Geometry check sheet. Reference: the model listing, model coordinates, mm. Face numbers are marked on the shaded views. A direction names the side the tool comes from. Give positions to 0.01 mm unless a question says otherwise; leave off trailing zeros. Order: outer loops, then holes, each group sorted by start corner. A loop starts at its lowest first (then second) coordinate and runs counter-clockwise, first axis right, second up. Notation, with made-up numbers: M -10,36 L 44,36 A16 cw 44,42 Z; hole C 15,77.25 d5. An arc over 180 degrees is marked long. Answer as CSV lines item,"result". Start each with the question number.
Q1. Section check A-A, the plane y = 24.5. Record the boundary of the cut face in (x, z).
Q2. Go/stop test with flat-tipped pins: pin 1 (1.5 mm diameter, centred on y = 56.5, z = 43.5, fed in from -X); pin 2 (5 mm diameter, centred on x = -24, y = 23.5, fed in from -Z); pin 3 (3 mm diameter, centred on x = 53, y = 30.5, fed in from +Z). Record where each tip stops, or that it passes through.
Q3. Section check D-D, the plane y = 62. Record the boundary of the cut face in (x, z), then the cut area to 3 significant figures.
Q4. Section check B-B, the plane x = 23.5. Record the boundary of the cut face in (y, z), then the cut area to 3 significant figures.
Q5. Set-up check for the marked faces 1, 2 and 3: record each of +Z, -Z, +X, -X, +Y, -Y from which the full face is reachable in a straight line by a thin tool's end or side.
Q6. Thickness scan on line 1 (X direction, y = 8, z = 107); line 2 (Z direction, x = -91, y = 5); line 3 (X direction, y = 18, z = 128). Record the ranges inside material, lowest first.
Q7. Section check C-C, the plane z = 39.5. Record the boundary of the cut face in (x, y).
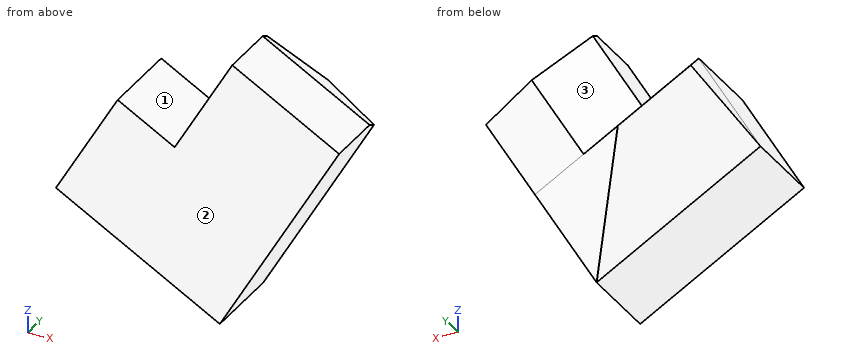
```python
from build123d import *

# Parameters (mm, degrees)
EXTRUDE1_DEPTH     = 50
EXTRUDE2_DEPTH     = 115
EXTRUDE3_DEPTH     = 105
CUT_EXTRUDE1_DEPTH = 155
CUT_EXTRUDE2_DEPTH = 75


with BuildPart() as part:
    # Sketch1 → Extrude1 (new body)
    with BuildSketch(Plane(origin=(0, 0, 0), x_dir=(1, 0, 0), z_dir=(0, 1, 0))):
        Polygon((0, 0), (72.5, -125.573683549), (7.548094716, -163.073683549), (-27.451905284, -102.451905284), (-62.092921435, -122.451905284), (-99.592921435, -57.5), align=None)
    extrude(amount=EXTRUDE1_DEPTH)

    # Sketch2 → Extrude2 (add)
    with BuildSketch(Plane(origin=(-99.592921435, 0, 57.5), x_dir=(0.5, 0, 0.866025404), z_dir=(-0.866025404, 0, 0.5))):
        Polygon((75, 50), (0, 50), (37.5, 94.690759722), align=None)
    extrude(amount=-EXTRUDE2_DEPTH)

    # Sketch3 → Extrude3 (add)
    with BuildSketch(Plane(origin=(72.5, 0, 125.573683549), x_dir=(0.866025404, 0, -0.5), z_dir=(0.5, 0, 0.866025404))):
        Polygon((0, 50), (-75, 50), (-37.5, 76.257782683), align=None)
    extrude(amount=-EXTRUDE3_DEPTH)

    # Sketch4 → Cut-Extrude1 (cut)
    with BuildSketch(Plane(origin=(72.5, 0, 125.573683549), x_dir=(0.866025404, 0, -0.5), z_dir=(0.5, 0, 0.866025404))):
        Polygon((0, 50), (0, 113.526991311), (-90.725946016, 113.526991311), align=None)
    extrude(amount=-CUT_EXTRUDE1_DEPTH, mode=Mode.SUBTRACT)

    # Sketch5 → Cut-Extrude2 (cut)
    with BuildSketch(Plane(origin=(0, 0, 0), x_dir=(-0.5, 0, -0.866025404), z_dir=(0.866025404, 0, -0.5))):
        Polygon((-145, 35), (-97.861503451, 102.320749887), (-145, 102.320749887), align=None)
    extrude(amount=-CUT_EXTRUDE2_DEPTH, mode=Mode.SUBTRACT)


solid = part.part
```
Answer block:
1,outline,"M -99.59,57.5 L 0,0 L 72.5,125.57 L 7.55,163.07 L -27.45,102.45 L -62.09,122.45 Z"
2,pin 1,"stops at x = -66.24"
2,pin 2,"stops at z = 12.41"
2,pin 3,"stops at z = 137.7"
3,outline,"M -94.56,66.22 L -9.81,17.29 L 48.21,117.77 L 12.94,138.13 L -17.64,85.16 L -67.13,113.73 Z"
3,area,"7,860 mm2"
4,outline,"M 0,40.7 L 50,40.7 L 76.26,115.7 L 73.91,122.4 L 35,153.86 L 0,153.86 Z"
4,area,"6,950 mm2"
5,face 1,"+Z, +Y, -Y"
5,face 2,"+Z, -Z, +X, -X, -Y"
5,face 3,"+Z, +Y"
6,line 1,"x = -71.01 to -35.33, -24.83 to 61.78"
6,line 2,"z = 52.54 to 72.38"
6,line 3,"x = -12.7 to 68.3"
7,outline,"M -68.42,0 L 22.81,0 L 22.81,50 L -22.41,77.42 L -68.42,50 Z"
